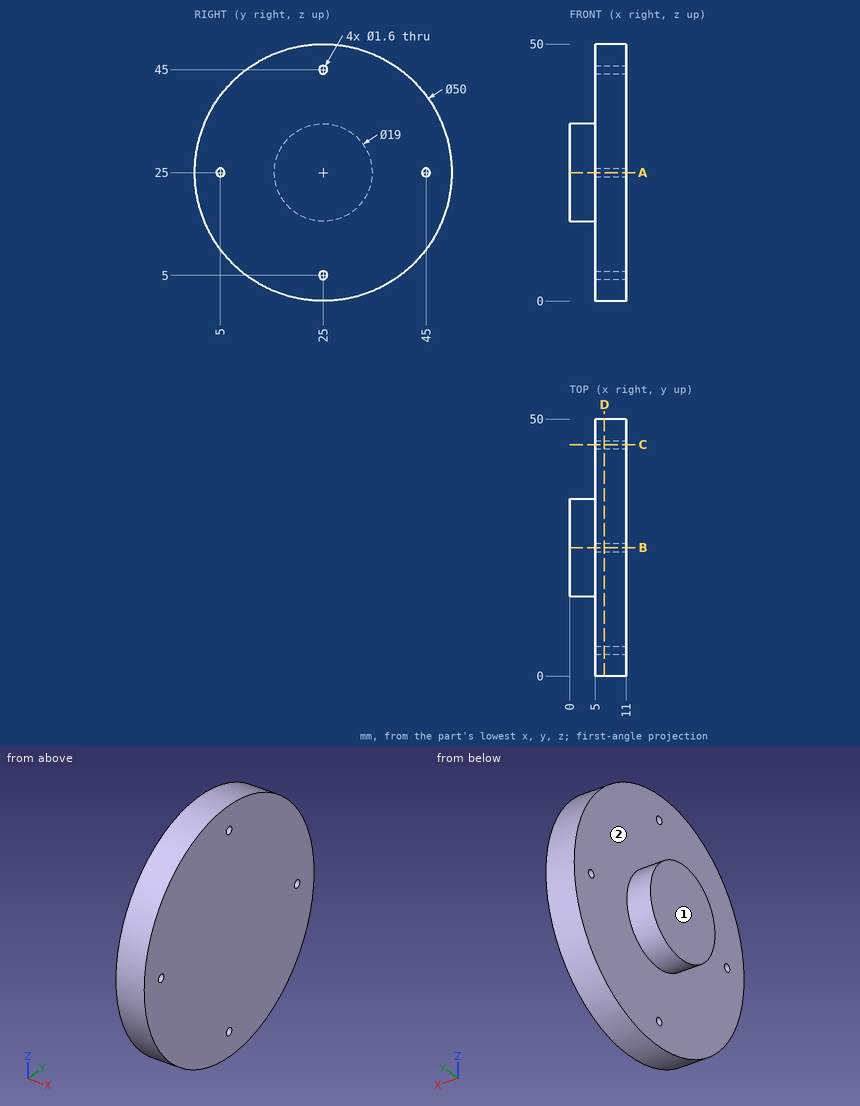
Verification items for this drawing (mm, ordinates from the low corner). A direction names the side the tool comes from. Give positions to 0.01 mm unless a question says otherwise; leave off trailing zeros. Loops run counter-clockwise (first coordinate to the right, second up) from the corner with the lowest first, then second, coordinate; pieces in that order, holes last.
(1) Set-up check for the marked faces 1 and 2: record each of +Z, -Z, +X, -X, +Y, -Y from which the full face is reachable in a straight line by a thin tool's end or side.
From the geometry:
face 1: +Z, -Z, -X, +Y, -Y
face 2: -X
(2) Depth check by flat-ended pin: pin 1 Ø1.4 at (y, z) = (25, 45) entering from -X; pin 2 Ø8 at (y, z) = (18.5, 42.5) entering from -X; pin 3 Ø2 at (x, z) = (5.5, 21.5) entering from -Y; pin 4 Ø6 at (x, z) = (3, 28) entering from -Y. Enter the tip coordinate at first touch or a pass-through.
From the geometry:
pin 1: passes through
pin 2: stops at x = 5
pin 3: stops at y = 0.13
pin 4: stops at y = 0.01
(3) Section check C-C on y = 45. Record the cut outline in (x, z).
From the geometry:
outline: (5, 10) - (11, 10) - (11, 24.2) - (5, 24.2) - close; (5, 25.8) - (11, 25.8) - (11, 40) - (5, 40) - close
(4) Thickness scan on L1, parallel to Y at x = 7.3, z = 25; L2, parallel to X at y = 12, z = 23; L3, parallel to Y at x = 7.85, z = 5. Record the ranges inside material, lowest first.
From the geometry:
L1: y = 0 to 4.2, 5.8 to 44.2, 45.8 to 50
L2: x = 5 to 11
L3: y = 10 to 24.2, 25.8 to 40
(5) Section check A-A on z = 25. Record the cut outline in (x, y).
From the geometry:
outline: (0, 15.5) - (5, 15.5) - (5, 5.8) - (11, 5.8) - (11, 44.2) - (5, 44.2) - (5, 34.5) - (0, 34.5) - close; (5, 0) - (11, 0) - (11, 4.2) - (5, 4.2) - close; (5, 45.8) - (11, 45.8) - (11, 50) - (5, 50) - close
(6) Section check D-D on x = 6.75. Record the cut outline in (y, z), then the cut area to 3 significant figures.
From the geometry:
outline: circle Ø50 at (25, 25); hole circle Ø1.6 at (5, 25); hole circle Ø1.6 at (25, 5); hole circle Ø1.6 at (25, 45); hole circle Ø1.6 at (45, 25)
area: 1,960 mm2
